```python
from build123d import *

# Parameters (mm, degrees)
SKETCH_1_R               = 10
EXTRUDE_1_DEPTH          = 10
SKETCH_2_W               = 27.353123027
SKETCH_2_H               = 11.793746162
CUT_EXTRUDE_1_DEPTH      = 10
CUT_EXTRUDE_1_DEPTH_BACK = 10
SKETCH_3_R               = 1.75
CUT_EXTRUDE_2_DEPTH      = 11
SKETCH_4_R               = 3
CUT_EXTRUDE_3_DEPTH      = 4
SKETCH_5_W               = 23.260827415
SKETCH_5_H               = 7
CUT_EXTRUDE_5_DEPTH      = 7
SKETCH_6_R               = 1.75
CUT_EXTRUDE_6_DEPTH      = 7


with BuildPart() as part:
    # Sketch 1 → Extrude 1 (new body)
    with BuildSketch(Plane(origin=(0, 0, 0), x_dir=(1, 0, 0), z_dir=(0, 1, 0))):
        Circle(SKETCH_1_R)
    extrude(amount=EXTRUDE_1_DEPTH)

    # Sketch 2 → Cut-Extrude 1 (cut, two sides)
    with BuildSketch(Plane(origin=(0, 0, 0), x_dir=(1, 0, 0), z_dir=(0, 1, 0))) as cut_extrude_1_sk:
        with Locations((1.294435554, -4.396873081)):
            Rectangle(SKETCH_2_W, SKETCH_2_H)
    extrude(amount=CUT_EXTRUDE_1_DEPTH, mode=Mode.SUBTRACT)
    extrude(cut_extrude_1_sk.sketch, amount=-CUT_EXTRUDE_1_DEPTH_BACK, mode=Mode.SUBTRACT)

    # Sketch 3 → Cut-Extrude 2 (cut, through all)
    with BuildSketch(Plane(origin=(0, 10, 0), x_dir=(1, 0, 0), z_dir=(0, 1, 0))):
        with Locations((0, 7)):
            Circle(SKETCH_3_R)
    extrude(amount=-CUT_EXTRUDE_2_DEPTH, mode=Mode.SUBTRACT)

    # Sketch 4 → Cut-Extrude 3 (cut)
    with BuildSketch(Plane(origin=(0, 10, 0), x_dir=(1, 0, 0), z_dir=(0, 1, 0))):
        Circle(SKETCH_4_R)
    extrude(amount=-CUT_EXTRUDE_3_DEPTH, mode=Mode.SUBTRACT)

    # Sketch 5 → Cut-Extrude 5 (cut)
    with BuildSketch(Plane.XZ):
        with Locations((0.625951198, -8)):
            Rectangle(SKETCH_5_W, SKETCH_5_H)
    extrude(amount=-CUT_EXTRUDE_5_DEPTH, mode=Mode.SUBTRACT)

    # Sketch 6 → Cut-Extrude 6 (cut)
    with BuildSketch(Plane.XY.offset(-1.5)):
        with Locations((-5, 3)):
            Circle(SKETCH_6_R)
        with Locations((5, 3)):
            Circle(SKETCH_6_R)
    extrude(amount=-CUT_EXTRUDE_6_DEPTH, mode=Mode.SUBTRACT)


solid = part.part
```
Geometry check sheet. Reference: the model listing, model coordinates, mm. A direction names the side the tool comes from. Give positions to 0.01 mm unless a question says otherwise; leave off trailing zeros. Order: outer loops, then holes, each group sorted by start corner. A loop starts at its lowest first (then second) coordinate and runs counter-clockwise, first axis right, second up. Notation, with made-up numbers: (-17.5, 70.5) - (-9.5, 70.5) arc R26 ccw to (-9.5, 91.5) - close; hole circle Ø10 at (22.25, 41). An arc over 180 degrees is marked (long way). Answer in a Markdown table with one row per item. Add a question column.
Q1. Cross-section at D-D, the plane z = -2. Enter the section's corners in (x, y).
Q2. Cross-section at A-A, the plane y = 3. Enter the section's corners in (x, z), then the cut area to 3 significant figures.
Q3. Tool access check on faces 1 (the flat face through (0, 3, -4.5)), 2 (the flat face through (0, 5, -1.5)). Record the directions out of +Z, -Z, +X, -X, +Y, -Y that give a thin tool (end or side, any length) a straight path to the whole face; none if there is none.
Q4. Cross-section at C-C, the plane y = 7.75. Enter the section's corners in (x, z), then the cut area to 3 significant figures.
Q5. Gauge pin test, flat ends, axial feed: pin 1 (3 mm diameter, centred on x = -1, z = -9, fed in from -Y); pin 2 (5 mm diameter, centred on y = 4, z = -4.5, fed in from +X); pin 3 (2 mm diameter, centred on x = 5, y = 3, fed in from +Z); pin 4 (2 mm diameter, centred on x = 1.5, y = 3, fed in from -Z). Record the tip position at first contact, or that the pin passes through.
Q6. Material ranges on probe 1 along Z at (x, y) = (0, 8.15); probe 2 along Y at (x, z) = (5, -2.6); probe 3 along Z at (x, y) = (1.25, 1.75), recorded low to high. Write a range as from..to.
Q7. Cross-section at B-B, the plane x = 5. Enter the section's corners in (y, z).
Q8. Mould release check, pull along Y, two halves, no side actions. Record for faces 3 (the cylindrical face through (3.61, 1.94, -2.98)), 4 (the cylindrical face through (0, 8, -3)), 5 (the flat face through (0, 6, -2)), 6 (the cylindrical face through (-5.38, 1.29, -2.98)): pulls with the +Y half, pulls with the -Y half, needs draft (parallel to the pull), parting line crosses it, or undercut.
Check values:
| question | item | result |
|---|---|---|
| 1 | outline | (-9.8, 0) - (9.8, 0) - (9.8, 10) - (2.24, 10) - (2.24, 6) - (-2.24, 6) - (-2.24, 10) - (-9.8, 10) - close; hole circle Ø3.5 at (-5, 3); hole circle Ø3.5 at (5, 3) |
| 2 | outline | (-9.89, -1.5) arc R10 ccw to (-8.93, -4.5) - (-6.75, -4.5) - (-6.75, -1.5) - close; (-3.25, -4.5) - (3.25, -4.5) - (3.25, -1.5) - (-3.25, -1.5) - close; (6.75, -4.5) - (8.93, -4.5) arc R10 ccw to (9.89, -1.5) - (6.75, -1.5) - close |
| 2 | area | 36.0 mm^2 |
| 3 | face 1 | -Z, +X, -X, -Y |
| 3 | face 2 | +Z, +X, -X, +Y, -Y |
| 4 | outline | (-9.89, -1.5) arc R10 ccw to (9.89, -1.5) - (2.6, -1.5) arc R3 cw to (-2.6, -1.5) - close; hole circle Ø3.5 at (0, -7) |
| 4 | area | 112 mm^2 |
| 5 | pin 1 | stops at y = 7 |
| 5 | pin 2 | stops at x = 9.8 |
| 5 | pin 3 | passes through |
| 5 | pin 4 | stops at z = -4.5 |
| 6 | probe 1 | z = -10..-8.75, -5.25..-3 |
| 6 | probe 2 | y = 0..1.25, 4.75..10 |
| 6 | probe 3 | z = -4.5..-1.5 |
| 7 | outline | (0, -4.5) - (1.25, -4.5) - (1.25, -1.5) - (0, -1.5) - close; (4.75, -4.5) - (7, -4.5) - (7, -8.66) - (10, -8.66) - (10, -1.5) - (4.75, -1.5) - close |
| 8 | face 3 | undercut |
| 8 | face 4 | needs draft |
| 8 | face 5 | pulls with the +Y half |
| 8 | face 6 | undercut |
